Verification items for the finished model (mm, model axes). Give positions to 0.01 mm unless a question says otherwise; leave off trailing zeros. Write each loop counter-clockwise with the first axis right and the second up, starting at its lowest first coordinate (ties: lowest second). Pieces come first, ordered by that corner, then holes.
from build123d import *

# Parameters (mm, degrees)
F0_R     = 0.5335
F0_R_2   = 0.36
F1_DEPTH = 35
F3_DEPTH = 0.5345
F4_DEPTH = 0.5345
F5_W     = 1.4
F5_H     = 0.65
F6_DEPTH = 1


with BuildPart() as f1:
    # F0 (on Right) → F1 (new body)
    with BuildSketch(Plane.YZ):
        Circle(F0_R)
        Circle(F0_R_2, mode=Mode.SUBTRACT)
    extrude(amount=F1_DEPTH)

    # F2 (on Front) → F3 (cut, through all)
    with BuildSketch(Plane.XZ):
        Polygon((3, -0.574455), (0, 0.53833), (0, -0.574455), align=None)
    extrude(amount=-F3_DEPTH, mode=Mode.SUBTRACT)

    # F2 (on Front) → F4 (cut, through all)
    with BuildSketch(Plane.XZ):
        Polygon((3, -0.574455), (0, 0.53833), (0, -0.574455), align=None)
    extrude(amount=F4_DEPTH, mode=Mode.SUBTRACT)

    # F5 (on Top) → F6 (cut)
    with BuildSketch(Plane.XY):
        with Locations((5.05, 0.046142)):
            Rectangle(F5_W, F5_H)
    extrude(amount=F6_DEPTH, mode=Mode.SUBTRACT)


solid = f1.part
Item 1: Scan lines: line 1 along Z through (x, y) = (15.5, 0); line 2 along Z through (x, y) = (14, -0.2). Record each from-to range of solid material in increasing order.
Answer key:
line 1: z = -0.53 to -0.36, 0.36 to 0.53
line 2: z = -0.49 to -0.3, 0.3 to 0.49
Item 2: Sectioned sample at A-A on x = 21. Record the cut outline in (y, z).
Answer key:
outline: circle Ø1.07 at (0, 0); hole circle Ø0.72 at (0, 0)
Item 3: Sectioned sample at B-B on y = 0. Record the cut outline in (x, z).
Answer key:
outline: (0.01, 0.53) - (0.48, 0.36) - (4.35, 0.36) - (4.35, 0.53) - close; (2.42, -0.36) - (2.89, -0.53) - (35, -0.53) - (35, -0.36) - close; (5.75, 0.36) - (35, 0.36) - (35, 0.53) - (5.75, 0.53) - close
